from build123d import *

# Parameters (mm, degrees)
SKETCH1_W           = 1219.2
SKETCH1_H           = 304.8
BOSS_EXTRUDE1_DEPTH = 304.8
CUT_EXTRUDE1_DEPTH  = 1294.156881434
CUT_EXTRUDE2_DEPTH  = 1294.156881434
CUT_EXTRUDE4_DEPTH  = 1294.156881434
SKETCH7_W           = 63.5
SKETCH7_H           = 279.4
CUT_EXTRUDE5_DEPTH  = 114.3


with BuildPart() as part:
    # Sketch1 → Boss-Extrude1 (new body)
    with BuildSketch(Plane(origin=(0, 0, 0), x_dir=(1, 0, 0), z_dir=(0, 1, 0))):
        with Locations((609.6, 152.4)):
            Rectangle(SKETCH1_W, SKETCH1_H)
    extrude(amount=-BOSS_EXTRUDE1_DEPTH)

    # Sketch2 → Cut-Extrude1 (cut, through all)
    with BuildSketch(Plane(origin=(0, 0, 0), x_dir=(1, 0, 0), z_dir=(0, 1, 0))):
        with BuildLine():
            Line((0, 260.35), (50.8, 260.35))
            ThreePointArc((50.8, 260.35), (57.15, 254), (50.8, 247.65))
            Line((50.8, 247.65), (0, 247.65))
            Line((0, 247.65), (0, 260.35))
        make_face()
        with BuildLine():
            Line((0, 57.15), (50.8, 57.15))
            ThreePointArc((50.8, 57.15), (57.15, 50.8), (50.8, 44.45))
            Line((50.8, 44.45), (0, 44.45))
            Line((0, 44.45), (0, 57.15))
        make_face()
        with BuildLine():
            Line((1219.2, 57.15), (1219.2, 44.45))
            Line((1219.2, 44.45), (1168.4, 44.45))
            ThreePointArc((1168.4, 44.45), (1162.05, 50.8), (1168.4, 57.15))
            Line((1168.4, 57.15), (1219.2, 57.15))
        make_face()
        with BuildLine():
            Line((1219.2, 260.35), (1219.2, 247.65))
            Line((1219.2, 247.65), (1168.4, 247.65))
            ThreePointArc((1168.4, 247.65), (1162.05, 254), (1168.4, 260.35))
            Line((1168.4, 260.35), (1219.2, 260.35))
        make_face()
        with BuildLine():
            Line((604.52, 304.8), (604.52, 254))
            ThreePointArc((604.52, 254), (610.235, 248.285), (615.95, 254))
            Line((615.95, 254), (615.95, 304.8))
            Line((615.95, 304.8), (604.52, 304.8))
        make_face()
        with BuildLine():
            Line((615.95, 0), (615.95, 50.8))
            ThreePointArc((615.95, 50.8), (610.235, 56.515), (604.52, 50.8))
            Line((604.52, 50.8), (604.52, 0))
            Line((604.52, 0), (615.95, 0))
        make_face()
    extrude(amount=-CUT_EXTRUDE1_DEPTH, mode=Mode.SUBTRACT)

    # Sketch4 → Cut-Extrude2 (cut, through all)
    with BuildSketch(Plane.ZY):
        Polygon((-304.8, -25.4), (-279.4, -25.4), (-264.757266468, -304.8), (-304.8, -304.8), align=None)
        Polygon((-40.042733532, -304.8), (-25.4, -25.4), (0, -25.4), (0, -304.8), align=None)
    extrude(amount=-CUT_EXTRUDE2_DEPTH, mode=Mode.SUBTRACT)

    # Sketch6 → Cut-Extrude4 (cut, through all)
    with BuildSketch(Plane.XY):
        Polygon((0, -25.4), (25.375259462, -25.4), (40.03808789, -304.8), (0, -304.8), align=None)
        Polygon((1193.8, -25.4), (1219.2, -25.4), (1219.2, -304.8), (1179.137171572, -304.8), align=None)
    extrude(amount=-CUT_EXTRUDE4_DEPTH, mode=Mode.SUBTRACT)

    # Sketch7 → Cut-Extrude5 (cut)
    with BuildSketch(Plane.XY):
        with Locations((1187.45, -165.1)):
            Rectangle(SKETCH7_W, SKETCH7_H)
        with Locations((31.75, -165.1)):
            Rectangle(SKETCH7_W, SKETCH7_H)
        with Locations((609.6, -165.1)):
            Rectangle(SKETCH7_W, SKETCH7_H)
    cut_extrude5 = extrude(amount=-CUT_EXTRUDE5_DEPTH, mode=Mode.SUBTRACT)

    # Mirror1: Cut-Extrude5 across plane
    add(cut_extrude5.mirror(Plane(origin=(0, 0, -152.4), x_dir=(1, 0, 0), z_dir=(0, 0, -1))), mode=Mode.SUBTRACT)


solid = part.part
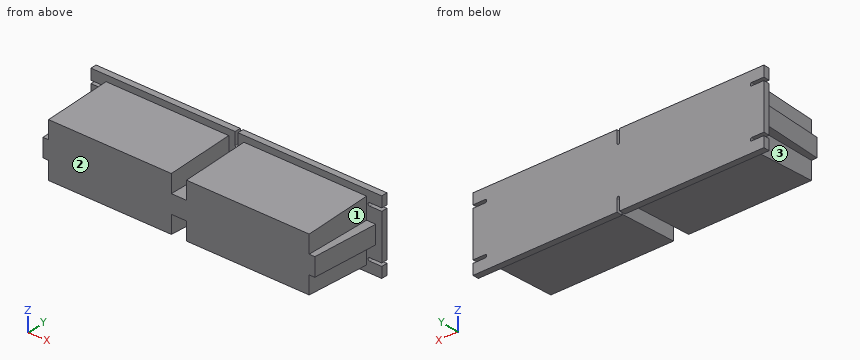
Part model, mm, in its own coordinate system. Face numbers are marked on the shaded views. A direction names the side the tool comes from. Give positions to 0.01 mm unless a question says otherwise; leave off trailing zeros. Order: outer loops, then holes, each group sorted by start corner. A loop starts at its lowest first (then second) coordinate and runs counter-clockwise, first axis right, second up. Notation, with made-up numbers: (35, 0) - (85, 0) arc R18 ccw to (85, 18) - close; hole circle Ø10 at (-24.75, 42.5). An arc over 180 degrees is marked (long way). Use a Markdown table: item, result.
1) Probe L1, parallel to X at y = -236, z = -88.5; L2, parallel to Y at x = 596, z = -278; L3, parallel to Z at x = 1072.5, y = -28. List the from-to ranges inside material, lowest first. Write a range as from..to.
Checked values:
| item | result |
|---|---|
| L1 | 63.5..577.85, 641.35..1155.7 |
| L2 | -25.4..0 |
| L3 | -279.26..-25.54 |
2) Saw through at D-D on y = -64. List the corners of the cut face in (x, z), plus the area to 3 significant figures.
Checked values:
| item | result |
|---|---|
| outline | (27.4, -190.5) - (63.5, -190.5) - (63.5, -277.38) - (577.85, -277.38) - (577.85, -190.5) - (641.35, -190.5) - (641.35, -277.38) - (1155.7, -277.38) - (1155.7, -190.5) - (1191.77, -190.5) - (1191.77, -114.3) - (1155.7, -114.3) - (1155.7, -27.42) - (641.35, -27.42) - (641.35, -114.3) - (577.85, -114.3) - (577.85, -27.42) - (63.5, -27.42) - (63.5, -114.3) - (27.4, -114.3) - close |
| area | 267,000 mm² |
3) Saw through at C-C on y = -143. List the corners of the cut face in (x, z).
Checked values:
| item | result |
|---|---|
| outline | (31.55, -190.5) - (63.5, -190.5) - (63.5, -273.24) - (577.85, -273.24) - (577.85, -190.5) - (641.35, -190.5) - (641.35, -273.24) - (1155.7, -273.24) - (1155.7, -190.5) - (1187.63, -190.5) - (1187.63, -114.3) - (1155.7, -114.3) - (1155.7, -31.56) - (641.35, -31.56) - (641.35, -114.3) - (577.85, -114.3) - (577.85, -31.56) - (63.5, -31.56) - (63.5, -114.3) - (31.55, -114.3) - close |
4) Saw through at B-B on z = -143. List the corners of the cut face in (x, y).
Checked values:
| item | result |
|---|---|
| outline | (0, -25.4) - (25.38, -25.4) - (40.04, -304.8) - (1179.14, -304.8) - (1193.8, -25.4) - (1219.2, -25.4) - (1219.2, 0) - (0, 0) - close |
5) Saw through at A-A on x = 76.5. List the corners of the cut face in (y, z).
Checked values:
| item | result |
|---|---|
| outline | (-304.8, -264.76) - (-25.4, -279.4) - (-25.4, -304.8) - (0, -304.8) - (0, 0) - (-25.4, 0) - (-25.4, -25.4) - (-304.8, -40.04) - close |
6) 3-axis set-ups, long thin cutter, end or side, ignore diameter. For the marked faces 1, 2 and 3: which of +Z, -Z, +X, -X, +Y, -Y reach the whole face in a straight line?
Checked values:
| item | result |
|---|---|
| face 1 | +Z, +X, -Y |
| face 2 | +Z, -Z, +X, -X, -Y |
| face 3 | -Z, -X, -Y |
7) Flat gauge pins, fed straight in: P1, Ø4, axis at x = 600.5, y = -150, coming from the +Z side; P2, Ø1, axis at y = -32.5, z = -73.5, coming from the +X side; P3, Ø10, axis at y = -198.5, z = -140, coming from the +X side. Where does each tip first touch, or does it go through?
Checked values:
| item | result |
|---|---|
| P1 | z = -114.3 |
| P2 | x = 1155.7 |
| P3 | x = 1184.98 |
